from build123d import *

# Parameters (mm, degrees)
SKETCH_2_W            = 7.400000122
SKETCH_2_H            = 11.88
SKETCH_2_R            = 0.6
EXTRUDE_1_DEPTH       = 6.05
SKETCH_3_W            = 7.400000122
SKETCH_3_H            = 5.56
EXTRUDE_2_DEPTH       = 5
CUT_EXTRUDE_1_DEPTH   = 3
CUT_EXTRUDE_START     = 3
CUT_EXTRUDE_2_DEPTH   = 3
SKETCH_7_R            = 0.6
CUT_EXTRUDE_2_2_DEPTH = 15.655173365
SKETCH_8_R            = 1
CUT_EXTRUDE_3_DEPTH   = 14.261301081
SKETCH_9_W            = 7.400000122
SKETCH_9_H            = 5.56
EXTRUDE_3_DEPTH       = 1


with BuildPart() as part:
    # Эскиз2 → Бобышка-Вытянуть1 (new body)
    with BuildSketch(Plane.XY):
        with Locations((-0.017150241, -0.38)):
            Rectangle(SKETCH_2_W, SKETCH_2_H)
        with Locations((-1.967150241, -5.12)):
            Circle(SKETCH_2_R, mode=Mode.SUBTRACT)
        with Locations((1.932849759, -5.12)):
            Circle(SKETCH_2_R, mode=Mode.SUBTRACT)
    extrude(amount=EXTRUDE_1_DEPTH)

    # Эскиз3 → Бобышка-Вытянуть2 (add)
    with BuildSketch(Plane.XY.offset(6.05)):
        with Locations((-0.017150241, 2.78)):
            Rectangle(SKETCH_3_W, SKETCH_3_H)
    extrude(amount=EXTRUDE_2_DEPTH)

    # Эскиз5 → Вырез-Вытянуть1 (cut)
    with BuildSketch(Plane(origin=(0, 5.56, 0), x_dir=(1, 0, 0), z_dir=(0, 1, 0))):
        with BuildLine():
            Line((-1.018455159, -10.651897729), (-1.374921155, -10.651897729))
            ThreePointArc((-1.374921155, -10.651897729), (-2.518455159, -8.551897729), (-1.374921155, -6.451897729))
            Line((-1.374921155, -6.451897729), (0.581544841, -6.451897729))
            Line((0.581544841, -6.451897729), (0.981544841, -6.451897729))
            Line((0.981544841, -6.451897729), (1.338010838, -6.451897729))
            ThreePointArc((1.338010838, -6.451897729), (2.481544841, -8.551897729), (1.338010838, -10.651897729))
            Line((1.338010838, -10.651897729), (-0.618455159, -10.651897729))
            Line((-0.618455159, -10.651897729), (-1.018455159, -10.651897729))
        make_face()
    extrude(amount=-CUT_EXTRUDE_1_DEPTH, mode=Mode.SUBTRACT)

    # Эскиз6 → Cut-Extrude 2 (cut)
    with BuildSketch(Plane(origin=(0, 2.56, 0), x_dir=(1, 0, 0), z_dir=(0, 1, 0)).offset(CUT_EXTRUDE_START)):
        with BuildLine():
            Line((-1.488149005, -11.051897729), (1.451238687, -11.051897729))
            ThreePointArc((1.451238687, -11.051897729), (2.881544841, -8.551897729), (1.451238687, -6.051897729))
            Line((1.451238687, -6.051897729), (-1.488149005, -6.051897729))
            ThreePointArc((-1.488149005, -6.051897729), (-2.918455159, -8.551897729), (-1.488149005, -11.051897729))
        make_face()
        with BuildLine():
            Line((-1.374921155, -10.651897729), (1.338010838, -10.651897729))
            ThreePointArc((1.338010838, -10.651897729), (2.481544841, -8.551897729), (1.338010838, -6.451897729))
            Line((1.338010838, -6.451897729), (-1.374921155, -6.451897729))
            ThreePointArc((-1.374921155, -6.451897729), (-2.518455159, -8.551897729), (-1.374921155, -10.651897729))
        make_face(mode=Mode.SUBTRACT)
    extrude(amount=-CUT_EXTRUDE_2_DEPTH, mode=Mode.SUBTRACT)

    # Эскиз7 → Cut-Extrude 2 2 (cut, through all)
    with BuildSketch(Plane(origin=(0, 2.56, 0), x_dir=(1, 0, 0), z_dir=(0, 1, 0))):
        with Locations(Location((-1.968455159, -8.551897729, 0), (0, 0, 270))):
            Circle(SKETCH_7_R)
        with Locations(Location((1.931544841, -8.551897729, 0), (0, 0, 270))):
            Circle(SKETCH_7_R)
    extrude(amount=-CUT_EXTRUDE_2_2_DEPTH, mode=Mode.SUBTRACT)

    # Эскиз8 → Вырез-Вытянуть3 (cut, through all)
    with BuildSketch(Plane(origin=(0, 0, 0), x_dir=(-1, 0, 0), z_dir=(0, 0, -1))):
        with Locations((0.017150241, -2.7)):
            Circle(SKETCH_8_R)
    extrude(amount=-CUT_EXTRUDE_3_DEPTH, mode=Mode.SUBTRACT)

    # Эскиз9 → Бобышка-Вытянуть3 (add)
    with BuildSketch(Plane.XY.offset(11.05)):
        with Locations((-0.017150241, 2.78)):
            Rectangle(SKETCH_9_W, SKETCH_9_H)
    extrude(amount=EXTRUDE_3_DEPTH)


solid = part.part
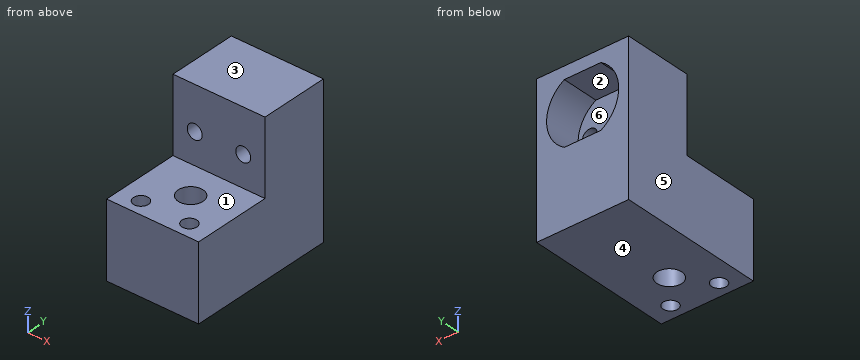
Work out the finished part from the listing and answer in its coordinate system (mm). Face numbers are marked on the shaded views. A direction names the side the tool comes from. Give positions to 0.01 mm unless a question says otherwise; leave off trailing zeros. Loops run counter-clockwise (first coordinate to the right, second up) from the corner with the lowest first, then second, coordinate; pieces in that order, holes last. Notation, with made-up numbers: (89.5, -9.5) -> (116.5, -9.5) arc R23 cw to (116.5, 21.5) -> close; hole circle Ø7 at (44, -12.5). An arc over 180 degrees is marked (long way). Use a Markdown table: item, result. Add a question column.
1) Consider line 1 along X through (y, z) = (-4.75, 2); line 2 along X through (y, z) = (-5.25, 4.75); line 3 along Z through (x, y) = (-0.5, 4.25). Determine where each line is inside the solid, lowest interval first.
2) For a pull along Z with two mould halves and no side action, classify the marked faces 4, 5 and 6 as +Z half, -Z half, draft (parallel to the pull), parting line (faces both ways), or undercut.
3) The part is cut by section D-D, the plane y = -2.7. Determine the outline of the cut face in (x, z).
4) The part is cut by section A-A, the plane y = -5.12. Determine the outline of the cut face in (x, z), plus the area to 4 significant figures.
5) Which of the six approach directions +Z, -Z, +X, -X, +Y, -Y give full straight-line access (tool end or side, diameter ignored) to the marked faces 1, 2 and 3?
6) The part is cut by section B-B, the plane z = 4. Determine the outline of the cut face in (x, y), plus the area to 3 significant figures.
7) The part is cut by section C-C, the plane x = 0.5. Determine the outline of the cut face in (y, z), plus the area to 3 significant figures.
8) Each of these flat-tipped pins is pushed along its axis until it touches: P1, Ø1.1, axis at x = 1.93, z = 8.55, coming from the +Y side; P2, Ø2, axis at x = -1.5, z = 10.5, coming from the -Y side; P3, Ø1.4, axis at x = 1.93, y = -5.12, coming from the -Z side; P4, Ø1.6, axis at x = -1.97, y = -5.12, coming from the +Z side. Where does it stop, or does it pass through?
Reported:
| question | item | result |
|---|---|---|
| 1 | line 1 | x = -3.72 to -2.44, -1.49 to 1.46, 2.41 to 3.68 |
| 1 | line 2 | x = -3.72 to -2.55, -1.38 to 1.35, 2.52 to 3.68 |
| 1 | line 3 | z = 0 to 6.05, 11.05 to 12.05 |
| 2 | face 4 | -Z half |
| 2 | face 5 | draft |
| 2 | face 6 | undercut |
| 3 | outline | (-3.72, 0) -> (-1.02, 0) -> (-1.02, 6.05) -> (-3.72, 6.05) -> close; (0.98, 0) -> (3.68, 0) -> (3.68, 6.05) -> (0.98, 6.05) -> close |
| 4 | outline | (-3.72, 0) -> (-2.57, 0) -> (-2.57, 6.05) -> (-3.72, 6.05) -> close; (-1.37, 0) -> (1.33, 0) -> (1.33, 6.05) -> (-1.37, 6.05) -> close; (2.53, 0) -> (3.68, 0) -> (3.68, 6.05) -> (2.53, 6.05) -> close |
| 4 | area | 30.25 mm^2 |
| 5 | face 1 | +Z, +X, -X, -Y |
| 5 | face 2 | +Y |
| 5 | face 3 | +Z, +X, -X, +Y, -Y |
| 6 | outline | (-3.72, -6.32) -> (3.68, -6.32) -> (3.68, 5.56) -> (-3.72, 5.56) -> close; hole circle Ø1.2 at (-1.97, -5.12); hole circle Ø2 at (-0.02, -2.7); hole circle Ø1.2 at (1.93, -5.12) |
| 6 | area | 82.5 mm^2 |
| 7 | outline | (-6.32, 0) -> (-3.56, 0) -> (-3.56, 6.05) -> (-6.32, 6.05) -> close; (-1.84, 0) -> (5.56, 0) -> (5.56, 6.05) -> (2.56, 6.05) -> (2.56, 11.05) -> (5.56, 11.05) -> (5.56, 12.05) -> (0, 12.05) -> (0, 6.05) -> (-1.84, 6.05) -> close |
| 7 | area | 79.9 mm^2 |
| 8 | P1 | passes through |
| 8 | P2 | stops at y = 0 |
| 8 | P3 | stops at z = 0 |
| 8 | P4 | stops at z = 6.05 |
